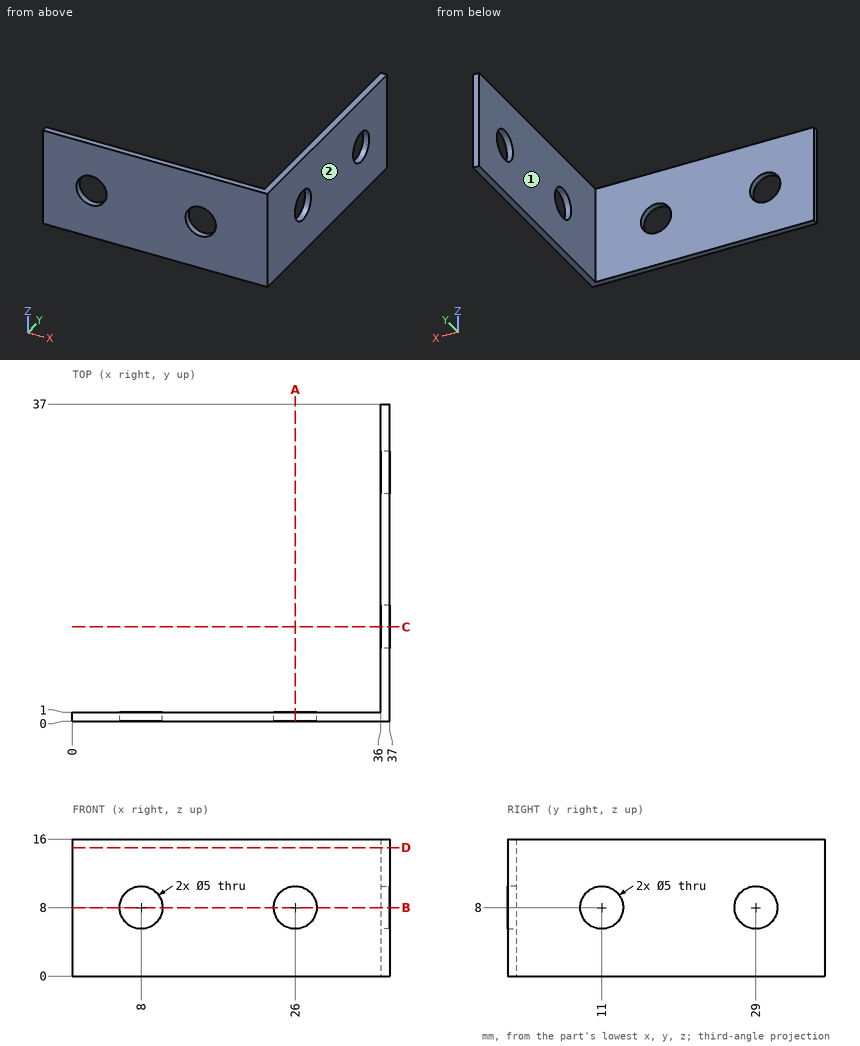
The figure shows three views and two pictorial views of one solid part (mm, origin at its lowest corner). Answer the questions. A direction names the side the tool comes from. Give positions to 0.01 mm unless a question says otherwise; leave off trailing zeros. Write each loop counter-clockwise with the first axis right and the second up, starting at its lowest first coordinate (ties: lowest second). Pieces come first, ordered by that corner, then holes. Notation, with made-up numbers: (15, 7) -> (67, 7) arc R18 cw to (67, 16) -> close; hole circle Ø3 at (-22.75, -0.75). An arc over 180 degrees is marked (long way). Write each question's results on one line, items separated by ' | '.
1. Find section C-C on y = 11. Determine the outline of the cut face in (x, z).
Data:
outline: (36, 0) -> (37, 0) -> (37, 5.5) -> (36, 5.5) -> close; (36, 10.5) -> (37, 10.5) -> (37, 16) -> (36, 16) -> close
2. Find section B-B on z = 8. Determine the outline of the cut face in (x, y).
Data:
outline: (0, 0) -> (5.5, 0) -> (5.5, 1) -> (0, 1) -> close; (10.5, 0) -> (23.5, 0) -> (23.5, 1) -> (10.5, 1) -> close; (28.5, 0) -> (37, 0) -> (37, 8.5) -> (36, 8.5) -> (36, 1) -> (28.5, 1) -> close; (36, 13.5) -> (37, 13.5) -> (37, 26.5) -> (36, 26.5) -> close; (36, 31.5) -> (37, 31.5) -> (37, 37) -> (36, 37) -> close
3. Straight lines are drawn through the part: L1, parallel to X at y = 0.4, z = 8; L2, parallel to Y at x = 24.5, z = 5.75; L3, parallel to X at y = 29, z = 3. For each, find the intervals that lie inside material, in ascending order.
Data:
L1: 0 to 5.5, 10.5 to 23.5, 28.5 to 37 | L2: 0 to 1 | L3: 36 to 37
4. Each of these flat-tipped pins is pushed along its axis until it touches: pin 1 Ø3 at (x, z) = (33, 13.5) entering from +Y; pin 2 Ø6 at (y, z) = (20.5, 8.5) entering from -X. Where does it stop, or does it pass through?
Data:
pin 1: y = 1 | pin 2: x = 36
5. A tool of negligible diameter and unlimited length cuts with its end or side. For the marked faces 1 and 2, from which of +Z, -Z, +X, -X, +Y, -Y can it reach the whole face along a straight path? Write none if from no direction.
Data:
face 1: +Z, -Z, -X, +Y | face 2: +Z, -Z, +X, +Y, -Y
6. Find section A-A on x = 26. Determine the outline of the cut face in (y, z), and give its area (3 significant figures).
Data:
outline: (0, 0) -> (1, 0) -> (1, 5.5) -> (0, 5.5) -> close; (0, 10.5) -> (1, 10.5) -> (1, 16) -> (0, 16) -> close | area: 11.0 mm^2
7. Find section D-D on z = 15. Determine the outline of the cut face in (x, y).
Data:
outline: (0, 0) -> (37, 0) -> (37, 37) -> (36, 37) -> (36, 1) -> (0, 1) -> close
